The drawing under review shows one solid part. Ordinate dimensions are in mm from its lowest x, y, z. Give positions to 0.01 mm unless a question says otherwise; leave off trailing zeros. Write each loop counter-clockwise with the first axis right and the second up, starting at its lowest first coordinate (ties: lowest second). Pieces come first, ordered by that corner, then holes. Notation, with made-up numbers: M 63.5,13 L 80.5,13 A34 cw 80.5,52 Z; hole C 69.25,-27.75 d9. An arc over 180 degrees is marked long. One line per item, written item: value. Start each with the question number.
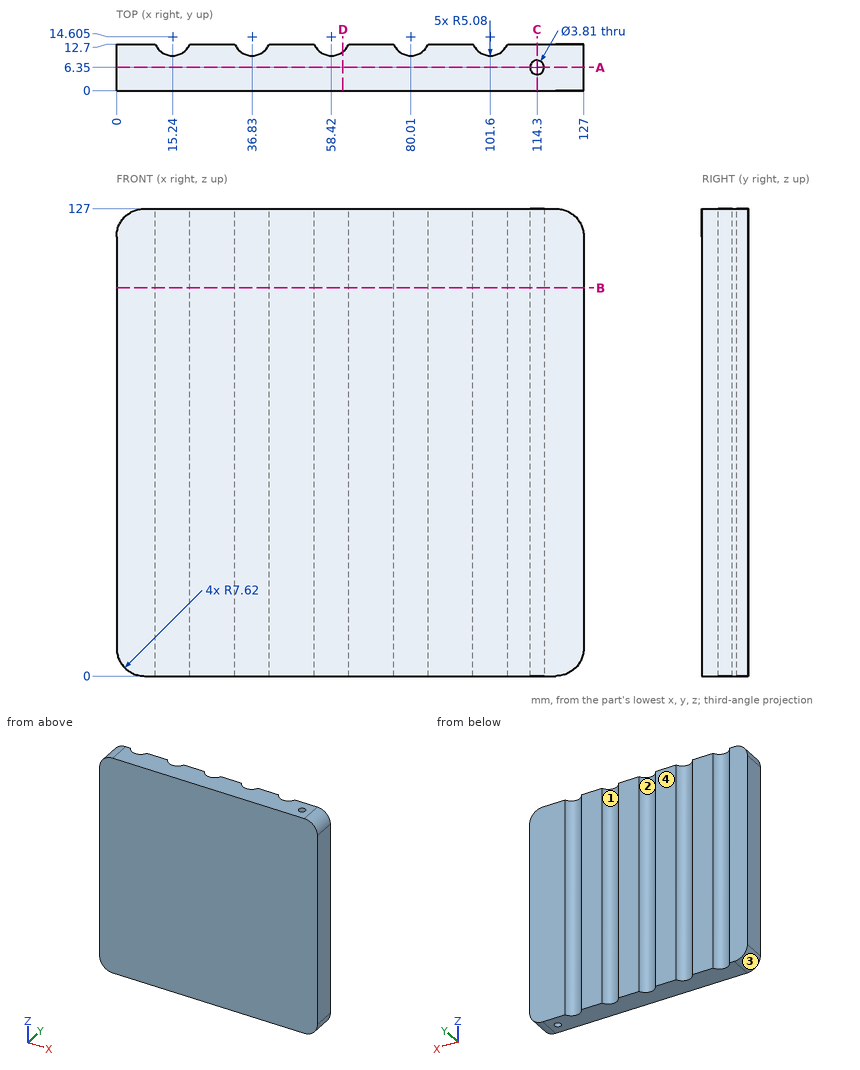
Q1. For P1, Ø1.5, axis at x = 15.5, z = 108.5, coming from the +Y side; P2, Ø2.5, axis at x = 114.3, y = 6.35, coming from the -Z side; P3, Ø4, axis at x = 79, z = 50, coming from the +Y side, all flat-tipped, find the tip position at first contact; note any pin that passes through.
Q2. Take a section at D-D, the plane x = 61.5. Give the boundary of the cut face in (y, z).
Q3. Wall thickness on line 1 (Y direction, x = 114.3, z = 81) (3 decimals); line 2 (Y direction, x = 114.5, z = 89); line 3 (X direction, y = 6.75, z = 122): over which ranges is each line inside the solid? List them lowest first. Write a range as from..to.
Q4. Take a section at C-C, the plane x = 114.3. Give the boundary of the cut face in (y, z) (3 decimals).
Q5. Take a section at A-A, the plane y = 6.35. Give the boundary of the cut face in (x, z) (3 decimals).
Q6. Take a section at B-B, the plane z = 105.5. Give the boundary of the cut face in (x, y) (3 decimals), then the cut area to 3 significant figures.
Q7. The part is to be moulded in two halves that separate along X. For the marked faces 1, 2, 3 and 4, say which applies: pulls with the +X half, pulls with the -X half, needs draft (parallel to the pull), parting line crosses it, or undercut.
Results list:
1. P1: stops at y = 9.63
1. P2: passes through
1. P3: stops at y = 10.51
2. outline: M 0,0 L 10.57,0 L 10.57,127 L 0,127 Z
3. line 1: y = 0..4.445, 8.255..12.7
3. line 2: y = 0..4.46, 8.24..12.7
3. line 3: x = 0.46..112.44, 116.16..126.54
4. outline: M 0,0 L 4.445,0 L 4.445,127 L 0,127 Z; M 8.255,0 L 12.7,0 L 12.7,127 L 8.255,127 Z
5. outline: M 0,7.62 A7.62 ccw 7.62,0 L 112.395,0 L 112.395,127 L 7.62,127 A7.62 ccw 0,119.38 Z; M 116.205,0 L 119.38,0 A7.62 ccw 127,7.62 L 127,119.38 A7.62 ccw 119.38,127 L 116.205,127 Z
6. outline: M 0,0 L 127,0 L 127,12.7 L 106.309,12.7 A5.08 cw 96.891,12.7 L 84.719,12.7 A5.08 cw 75.301,12.7 L 63.129,12.7 A5.08 cw 53.711,12.7 L 41.539,12.7 A5.08 cw 32.121,12.7 L 19.949,12.7 A5.08 cw 10.531,12.7 L 0,12.7 Z; hole C 114.3,6.35 d3.81
6. area: 1,490 mm^2
7. face 1: undercut
7. face 2: undercut
7. face 3: pulls with the -X half
7. face 4: needs draft
